Build history of the part. All positions in model axes, mm. A direction names the side the tool comes from. Give positions to 0.01 mm unless a question says otherwise; leave off trailing zeros. Write each loop counter-clockwise with the first axis right and the second up, starting at its lowest first coordinate (ties: lowest second). Pieces come first, ordered by that corner, then holes. Notation, with made-up numbers: (74.5, 21.5) -> (93.5, 21.5) arc R24 ccw to (93.5, 40.5) -> close; hole circle Ø2 at (65.25, 2). An arc over 180 degrees is marked (long way). Put each result on its own line as item: value. Start each with the question number.
Item 1: Two-plate mould, pull along Y, no slides. Class faces 1 (the flat face through (-13, 9.525, 38)), 2 (the flat face through (-5, 1.3, 77.47)), 3 (the flat face through (-12, 0, 1.27)), 4 (the flat face through (-5, 0, 87.757)): pulls with the +Y half, pulls with the -Y half, needs draft (parallel to the pull), parting line crosses it, or undercut.
Item 2: Slice it at D-D, the plane y = -7. List the corners of the cut face in (x, z), plus the area to 3 significant figures.
Item 3: Slice it at B-B, the plane x = -9.5. List the corners of the cut face in (y, z) (1 decimal), plus the area to 3 significant figures.
Item 4: Drill centre lines: line 1 along Y through (x, z) = (-7.5, 17) (3 decimals); line 2 along Z through (x, y) = (-3.25, 5.75); line 3 along Y through (x, z) = (-13.25, 74) (3 decimals). Where is each one in solid material? Low to high.
Item 5: Tool access for faces 5 (the flat face through (-12, -8.89, 74)), 6 (the flat face through (-12, 0, 76.2)), 7 (the flat face through (-10, -1.588, 84.2)), 8 (the flat face through (-3, 3.433, 81)): list every direction of +Z, -Z, +X, -X, +Y, -Y with a clear straight run to the whole face (end or side of a thin tool).
Item 6: Slice it at C-C, the plane z = 66. Give the number of separate pieces and of enclosed holes in the cut face, plus the area to 3 significant figures.
Item 7: Flat gauge pins, fed straight in: pin 1 Ø8 at (y, z) = (6.5, 28.5) entering from -X; pin 2 Ø4 at (y, z) = (-1.5, 77) entering from -X; pin 3 Ø0.7 at (x, y) = (-2.5, -9.5) entering from +Z; pin 4 Ø1.9 at (x, z) = (-5, 80) entering from -Y. Where does each tip first touch, or does it go through?
```python
from build123d import *

# Parameters (mm, degrees)
F1_DEPTH  = 76.2
F2_T      = -1.27
F4_DEPTH  = 76.2
F6_DEPTH  = 12.7
F8_DEPTH  = 1.27
F10_DEPTH = 1.27
F12_DEPTH = 1.5875
F13_W     = 6.6033280455
F13_H     = 6.9497893564
F13_W_2   = 5.3267844487
F13_H_2   = 5.3683998995
F14_DEPTH = 6.35
F15_W     = 2.0411710721
F15_H     = 2.829067409
F15_W_2   = 2.1245945245
F15_H_2   = 2.8308555484
F16_DEPTH = 0.635
F17_W     = 2.6483945549
F17_H     = 2.4718344212
F17_W_2   = 2.1775695495
F17_H_2   = 2.236418426
F18_DEPTH = 0.635


# Not quite as in the source:
# - a feature names something its author has since deleted; it is built from what else it names


with BuildPart() as f1:
    # F0 (on Top) → F1 (new body)
    with BuildSketch(Plane.XY):
        with BuildLine():
            Line((0, -9.525), (0, 9.525))
            Line((0, 9.525), (-25.4, 9.525))
            Line((-25.4, 9.525), (-25.4, 9.4535289675))
            ThreePointArc((-25.4, 9.4535289675), (-22.0324039546, 8.0586250129), (-20.6375, 4.6910289675))
            ThreePointArc((-20.6375, 4.6910289675), (-21.7533513451, 1.6278019374), (-24.5780185671, 0))
            ThreePointArc((-24.5780185671, 0), (-21.7533513451, -1.6278019374), (-20.6375, -4.6910289675))
            ThreePointArc((-20.6375, -4.6910289675), (-22.0324039546, -8.0586250129), (-25.4, -9.4535289675))
            Line((-25.4, -9.4535289675), (-25.4, -9.525))
            Line((-25.4, -9.525), (0, -9.525))
        make_face()
    extrude(amount=F1_DEPTH)

    # F2
    f2_openings = [f1.faces().sort_by_distance(p)[0] for p in [
        (-10.85856, 0, 76.2),
    ]]
    offset(amount=F2_T, openings=f2_openings)

    # F3 (on Top) → F4 (join)
    with BuildSketch(Plane.XY):
        with BuildLine():
            Line((-1.27, 1.8135049587), (-1.27, 2.6920572227))
            ThreePointArc((-1.27, 2.6920572227), (-3.9620572227, 0), (-1.27, -2.6920572227))
            Line((-1.27, -2.6920572227), (-1.27, -1.8135049587))
            ThreePointArc((-1.27, -1.8135049587), (-3.0835049587, 0), (-1.27, 1.8135049587))
        make_face()
    extrude(amount=F4_DEPTH)

    # F5 (on face) → F6 (cut)
    with BuildSketch(Plane(origin=(-1.27, 0, 0), x_dir=(0, -1, 0), z_dir=(-1, 0, 0))):
        Polygon((-2.6920572227, 1.27), (2.6920572227, 1.27), (2.6920572227, 10.6323556975), (-3.4403376048, 10.6323556975), (-3.4403376048, 1.27), align=None)
    extrude(amount=F6_DEPTH, mode=Mode.SUBTRACT)

    # F7 (on face) → F8 (join)
    with BuildSketch(Plane.XY.offset(76.2)):
        with BuildLine():
            Line((0, -9.525), (0, 9.525))
            Line((0, 9.525), (-25.4, 9.525))
            Line((-25.4, 9.525), (-25.4, 9.4535289675))
            ThreePointArc((-25.4, 9.4535289675), (-20.6554014022, 5.1035703547), (-24.5780185671, 0))
            ThreePointArc((-24.5780185671, 0), (-20.6554014022, -5.1035703547), (-25.4, -9.4535289675))
            Line((-25.4, -9.4535289675), (-25.4, -9.525))
            Line((-25.4, -9.525), (0, -9.525))
        make_face()
        with BuildLine():
            ThreePointArc((-1.27, 2.6920572227), (-3.9620572227, 0), (-1.27, -2.6920572227))
            Line((-1.27, -2.6920572227), (-1.27, -8.255))
            Line((-1.27, -8.255), (-20.5328481912, -8.255))
            ThreePointArc((-20.5328481912, -8.255), (-19.4179492319, -3.9124887578), (-21.6072037392, 0))
            ThreePointArc((-21.6072037392, 0), (-19.4179492319, 3.9124887578), (-20.5328481912, 8.255))
            Line((-20.5328481912, 8.255), (-1.27, 8.255))
            Line((-1.27, 8.255), (-1.27, 2.6920572227))
        make_face(mode=Mode.SUBTRACT)
        with BuildLine():
            ThreePointArc((-1.27, -1.8135049587), (-3.0835049587, 0), (-1.27, 1.8135049587))
            Line((-1.27, 1.8135049587), (-1.27, -1.8135049587))
        make_face(mode=Mode.SUBTRACT)
        with BuildLine():
            Line((-1.27, -8.255), (-1.27, -2.6920572227))
            ThreePointArc((-1.27, -2.6920572227), (-3.9620572227, 0), (-1.27, 2.6920572227))
            Line((-1.27, 2.6920572227), (-1.27, 8.255))
            Line((-1.27, 8.255), (-20.5328481912, 8.255))
            ThreePointArc((-20.5328481912, 8.255), (-19.4179492319, 3.9124887578), (-21.6072037392, 0))
            ThreePointArc((-21.6072037392, 0), (-19.4179492319, -3.9124887578), (-20.5328481912, -8.255))
            Line((-20.5328481912, -8.255), (-1.27, -8.255))
        make_face()
    extrude(amount=F8_DEPTH)

    # F9 (on face) → F10 (cut)
    with BuildSketch(Plane.XY.offset(77.47)):
        with BuildLine():
            ThreePointArc((-1.8017621012, -1.7337904437), (-3.0835049587, 0), (-1.8017621012, 1.7337904437))
            ThreePointArc((-1.8017621012, 1.7337904437), (-5.239634374, 0), (-1.8017621012, -1.7337904437))
        make_face()
        with BuildLine():
            ThreePointArc((-1.27, -1.1662306034), (-1.0148042261, -0.6077592736), (-0.9273755434, 0))
            ThreePointArc((-0.9273755434, 0), (-1.0148042261, 0.6077592736), (-1.27, 1.1662306034))
            Line((-1.27, 1.1662306034), (-1.27, -1.1662306034))
        make_face()
        with BuildLine():
            Line((-1.27, -1.1662306034), (-1.27, 1.1662306034))
            ThreePointArc((-1.27, 1.1662306034), (-1.5100785054, 1.4741856232), (-1.8017621012, 1.7337904437))
            ThreePointArc((-1.8017621012, 1.7337904437), (-3.0835049587, 0), (-1.8017621012, -1.7337904437))
            ThreePointArc((-1.8017621012, -1.7337904437), (-1.5100785054, -1.4741856232), (-1.27, -1.1662306034))
        make_face()
    extrude(amount=-F10_DEPTH, mode=Mode.SUBTRACT)

    # F11 (on Front) → F12 (join, symmetric)
    with BuildSketch(Plane.XZ):
        Polygon((-7.4378219433, 87.7572894096), (-17.725111353, 77.47), (-16.455111353, 77.47), (-7.4378219433, 86.4872894096), (-2.1149073727, 86.4872894096), (-2.1149073727, 87.7572894096), align=None)
    extrude(amount=F12_DEPTH, both=True)

    # F13 (on face) → F14 (join)
    with BuildSketch(Plane.XY.offset(77.47)):
        with Locations((-3.3016640227, -0.0416187104)):
            Rectangle(F13_W, F13_H)
        with Locations((-3.1908567762, 0.0832278747)):
            Rectangle(F13_W_2, F13_H_2, mode=Mode.SUBTRACT)
    extrude(amount=F14_DEPTH)

    # F15 (on face) → F16 (cut)
    with BuildSketch(Plane(origin=(0, 9.525, 0), x_dir=(-1, 0, 0), z_dir=(0, 1, 0))):
        with Locations((2.4719407083, 74.3873603642)):
            Rectangle(F15_W, F15_H)
        with Locations((11.8596078828, 73.9940367639)):
            Rectangle(F15_W_2, F15_H_2)
    extrude(amount=-F16_DEPTH, mode=Mode.SUBTRACT)

    # F17 (on face) → F18 (cut)
    with BuildSketch(Plane.XZ.offset(9.525)):
        with Locations((-12.3509913683, 74.2306262255)):
            Rectangle(F17_W, F17_H)
        with Locations((-2.5225046556, 74.5248906314)):
            Rectangle(F17_W_2, F17_H_2)
    extrude(amount=-F18_DEPTH, mode=Mode.SUBTRACT)


solid = f1.part
```
Values follow:
1. face 1: pulls with the +Y half
1. face 2: undercut
1. face 3: undercut
1. face 4: needs draft
2. outline: (-21.23, 0) -> (0, 0) -> (0, 77.47) -> (-21.23, 77.47) -> close; hole (-19.83, 1.27) -> (-1.27, 1.27) -> (-1.27, 76.2) -> (-19.83, 76.2) -> close
2. area: 255 mm2
3. outline: (-9.5, 0) -> (9.5, 0) -> (9.5, 77.5) -> (-9.5, 77.5) -> close; (-1.6, 84.4) -> (1.6, 84.4) -> (1.6, 85.7) -> (-1.6, 85.7) -> close; hole (-8.3, 1.3) -> (8.3, 1.3) -> (8.3, 76.2) -> (-8.3, 76.2) -> close
3. area: 243 mm2
4. line 1: -9.525 to -8.255, 8.255 to 9.525
4. line 2: 0 to 1.27, 76.2 to 77.47
4. line 3: -8.89 to -8.255, 8.255 to 9.525
5. face 5: -Y
5. face 6: none
5. face 7: +Z, -X, -Y
5. face 8: +Z, +X, -X, +Y
6. separate pieces: 1
6. enclosed holes: 2
6. area: 111 mm2
7. pin 1: x = -25.4
7. pin 2: x = -24.58
7. pin 3: z = 77.47
7. pin 4: y = -3.52
